For this review, take the finished solid that the model builds, in its own axes (mm). A direction names the side the tool comes from. Round coordinates to 2 decimals unless told otherwise and drop trailing zeros. Order: outer loops, then holes, each group sorted by start corner. A loop starts at its lowest first (then second) coordinate and runs counter-clockwise, first axis right, second up. Notation, with made-up numbers: (-18, 85.25) - (-10, 85.25) arc R20 cw to (-10, 100.25) - close; hole circle Ø2 at (27.5, 40.5). An arc over 180 degrees is marked (long way). One line per item, written item: value.
```python
from build123d import *

# Parameters (mm, degrees)
SKETCH_1_W          = 36
SKETCH_1_H          = 20
EXTRUDE_1_DEPTH     = 3
SKETCH_6_R          = 1.25
CUT_EXTRUDE_3_DEPTH = 42.291645644
EXTRUDE_2_DEPTH     = 20
CUT_EXTRUDE_1_REACH = 49.17
SKETCH_3_R          = 5
CUT_EXTRUDE_2_DEPTH = 43.766809561
FILLET_1_R          = 2
FILLET_3_R          = 3
FILLET_4_R          = 2


with BuildPart() as part:
    # 草图1 → 凸台-拉伸1 (new body)
    with BuildSketch(Plane(origin=(0, 0, 0), x_dir=(1, 0, 0), z_dir=(0, 1, 0))):
        with Locations((18, 10)):
            Rectangle(SKETCH_1_W, SKETCH_1_H)
    extrude(amount=EXTRUDE_1_DEPTH)

    # 草图6 → 切除-拉伸3 (cut, through all)
    with BuildSketch(Plane(origin=(0, 3, 0), x_dir=(1, 0, 0), z_dir=(0, 1, 0))):
        with Locations(Location((3, 3, 0), (0, 0, 270))):
            Circle(SKETCH_6_R)
        with Locations(Location((3, 17, 0), (0, 0, 270))):
            Circle(SKETCH_6_R)
        with Locations(Location((33, 17, 0), (0, 0, 270))):
            Circle(SKETCH_6_R)
        with Locations(Location((33, 3, 0), (0, 0, 270))):
            Circle(SKETCH_6_R)
    extrude(amount=-CUT_EXTRUDE_3_DEPTH, mode=Mode.SUBTRACT)

    # 草图2 → 凸台-拉伸2 (add)
    with BuildSketch(Plane(origin=(0, 3, 0), x_dir=(1, 0, 0), z_dir=(0, 1, 0))):
        Polygon((6, 0), (30, 0), (30, 16), (27.5, 16), (27.5, 3), (8.5, 3), (8.5, 16), (6, 16), align=None)
    extrude(amount=EXTRUDE_2_DEPTH)

    # 草图3 → 切除-拉伸1 (cut, up to next)
    with BuildSketch(Plane.XY, mode=Mode.PRIVATE) as cut_extrude_1_sk1:
        with Locations((18, 12.5)):
            Circle(SKETCH_3_R)
    cut_extrude_1_tool1 = extrude(cut_extrude_1_sk1.sketch, amount=-CUT_EXTRUDE_1_REACH, mode=Mode.PRIVATE) & part.part
    add(cut_extrude_1_tool1.solids().sort_by_distance((18, 12.5, 0))[0], mode=Mode.SUBTRACT)

    # 草图4 → 切除-拉伸2 (cut, through all)
    with BuildSketch(Plane(origin=(30, 0, 0), x_dir=(0, 0, -1), z_dir=(1, 0, 0))):
        Polygon((3, 23), (16, 23), (16, 3), align=None)
    extrude(amount=-CUT_EXTRUDE_2_DEPTH, mode=Mode.SUBTRACT)

    # 圆角1
    fillet_1_edges = [part.edges().sort_by_distance(p)[0] for p in [
        (0, 1.5, -20),
        (36, 1.5, -20),
        (36, 1.5, 0),
        (0, 1.5, 0),
    ]]
    fillet(fillet_1_edges, radius=FILLET_1_R)

    # 圆角3
    fillet_3_edges = [part.edges().sort_by_distance(p)[0] for p in [
        (28.75, 3, -16),
        (7.25, 3, -16),
    ]]
    fillet(fillet_3_edges, radius=FILLET_3_R)

    # 圆角4
    fillet_4_edges = [part.edges().sort_by_distance(p)[0] for p in [
        (30, 23, -1.5),
        (6, 23, -1.5),
    ]]
    fillet(fillet_4_edges, radius=FILLET_4_R)


solid = part.part
```
Item 1: For P1, Ø6, axis at x = 10, z = -9.5, coming from the +Y side; P2, Ø2, axis at x = 22, z = -12, coming from the +Y side; P3, Ø5.5, axis at y = 9.5, z = -9.5, coming from the +X side, all flat-tipped, find the tip position at first contact; note any pin that passes through.
Returned:
P1: y = 17
P2: y = 3
P3: x = 30
Item 2: Take a section at B-B (y = 2.25). Write out the cut boundary in (x, z).
Returned:
outline: (0, -18) arc R2 ccw to (2, -20) - (34, -20) arc R2 ccw to (36, -18) - (36, -2) arc R2 ccw to (34, 0) - (2, 0) arc R2 ccw to (0, -2) - close; hole circle Ø2.5 at (3, -17); hole circle Ø2.5 at (3, -3); hole circle Ø2.5 at (33, -17); hole circle Ø2.5 at (33, -3)
Item 3: Take a section at A-A (x = 33). Write out the cut boundary in (y, z), plus the area to 3 significant figures.
Returned:
outline: (0, -20) - (3, -20) - (3, -18.25) - (0, -18.25) - close; (0, -15.75) - (3, -15.75) - (3, -4.25) - (0, -4.25) - close; (0, -1.75) - (3, -1.75) - (3, 0) - (0, 0) - close
area: 45.0 mm^2
Item 4: The part is to be moulded in two halves that separate along X. For faces 4 (the flat face through (36, 1, -10)), 5 (the flat face through (8.5, 8, -7)), 6 (the flat face through (7.267, 13.552, -9.141)), say which applies: +X half, -X half, draft (parallel to the pull), parting line (faces both ways), or undercut.
Returned:
face 4: +X half
face 5: undercut
face 6: draft
Item 5: Take a section at C-C (z = -17). Write out the cut boundary in (x, y).
Returned:
outline: (0, 0) - (1.75, 0) - (1.75, 3) - (0, 3) - close; (4.25, 0) - (31.75, 0) - (31.75, 3) - (30, 3) - (30, 3.07) - (27.5, 3.07) - (27.5, 3) - (8.5, 3) - (8.5, 3.07) - (6, 3.07) - (6, 3) - (4.25, 3) - close; (34.25, 0) - (36, 0) - (36, 3) - (34.25, 3) - close
Item 6: Machinability: for faces 1 (the flat face through (18, 3, -10)), 2 (the cylindrical face through (2.521, 1.521, -15.845)), 3 (the flat face through (6, 10, -5)), which of the approach directions +Z, -Z, +X, -X, +Y, -Y give a long, thin tool a straight path to every point of the face, cutting with its end or side? Answer none if there is none.
Returned:
face 1: -Z, +Y
face 2: +Y, -Y
face 3: +Z, -Z, -X, +Y
Item 7: Wall thickness on line 1 (X direction, y = 2.2, z = -3); line 2 (X direction, y = 7, z = -7.5); line 3 (Y direction, x = 18, z = -1.25): over which ranges is each line inside the solid? List them lowest first.
Returned:
line 1: 0 to 1.75, 4.25 to 31.75, 34.25 to 36
line 2: 6 to 8.5, 27.5 to 30
line 3: 0 to 7.5, 17.5 to 23
Item 8: Take a section at D-D (x = 14.5). Write out the cut boundary in (y, z), plus the area to 3 significant figures.
Returned:
outline: (0, -20) - (3, -20) - (3, -3) - (8.93, -3) - (8.93, 0) - (0, 0) - close; (16.07, -3) - (23, -3) - (23, 0) - (16.07, 0) - close
area: 98.6 mm^2
